Solid Edge part; units mm, degrees
sketch "Sketch1" plane through (0, 0, 0) normal (0, 0, 1) x (1, 0, 0)
  circle A0 centre (0, 0) radius 11
extrude "Protrusion1" add sketch "Sketch1" along normal blind 28
sketch "Sketch2" plane through (0, 0, 28) normal (0, 0, 1) x (1, 0, 0)
  circle A0 centre (0, 0) radius 19
extrude "ExtrudedProtrusion_2" add sketch "Sketch2" along normal blind 4
sketch "Sketch3" plane through (0, 0, 32) normal (0, 0, 1) x (1, 0, 0)
  line L0 (14, 14) -> (14, -14)
  line L1 (14, -14) -> (-14, -14)
  line L2 (-14, -14) -> (-14, 14)
  line L3 (-14, 14) -> (14, 14)
extrude "ExtrudedProtrusion_3" add sketch "Sketch3" along normal blind 7.5
sketch "Sketch4" plane through (0, 0, 39.5) normal (0, 0, 1) x (1, 0, 0)
  circle A0 centre (0, 0) radius 7
extrude "ExtrudedProtrusion_4" add sketch "Sketch4" along normal blind 20
sketch "Sketch5" plane through (0, 0, 59.5) normal (0, 0, 1) x (1, 0, 0)
  line L0 (7, -25) -> (7, 7)
  line L1 (7, 7) -> (-7, 7)
  line L2 (-7, 7) -> (-7, -25)
  line L3 (-7, -25) -> (7, -25)
extrude "ExtrudedProtrusion_5" add sketch "Sketch5" against normal blind 3.5
sketch "Sketch6" plane through (0, -9, 59.5) normal (0, 0, 1) x (1, 0, 0)
  circle A0 centre (0, 9) radius 5
  circle A1 centre (0, 9) radius 4
extrude "ExtrudedProtrusion_6" add sketch "Sketch6" along normal blind 10
sketch "Sketch7" plane through (0, -12.5, 56) normal (0, 0, -1) x (0, -1, 0)
  line L0 (-5.4984, 7) -> (-5.4984, -7)
  line L1 (-5.4984, -7) -> (-19.5, -7)
  line L2 (-19.5, -7) -> (-19.5, 7)
  line L3 (-19.5, 7) -> (-5.4984, 7)
extrude "Protrusion2" add sketch "Sketch7" along normal blind 12
sketch "Sketch8" plane through (7, -9, 51.75) normal (1, 0, 0) x (0, 1, 0)
  circle A0 centre (9, -4.5) radius 6.75
extrude "ExtrudedProtrusion_10" add sketch "Sketch8" against normal blind 26
sketch "Sketch9" plane through (-19, 0, 47.25) normal (-1, 0, 0) x (0, -1, 0)
  circle A0 centre (0, 0) radius 10.5
extrude "ExtrudedProtrusion_11" add sketch "Sketch9" along normal blind 15
sketch "Sketch10" plane through (-34, 0, 47.25) normal (-1, 0, 0) x (0, -1, 0)
  circle A0 centre (0, 0) radius 8.5
extrude "ExtrudedCutout_1" cut sketch "Sketch10" against normal blind 12.1174
sketch "Sketch11" plane through (0, 0, 0) normal (0, 0, -1) x (-1, 0, 0)
  circle A0 centre (0, 0) radius 10
extrude "ExtrudedCutout_2" cut sketch "Sketch11" against normal blind 35.1549
sketch "Sketch12" plane through (0, -9, 59.5) normal (0, 0, 1) x (1, 0, 0)
  circle A0 centre (0, 9) radius 4
extrude "Cutout1" cut sketch "Sketch12" against normal blind 106.077
sketch "Sketch13" plane through (-21.8826, 0, 47.25) normal (-1, 0, 0) x (0, -1, 0)
  circle A0 centre (0, 0) radius 4
extrude "ExtrudedCutout_4" cut sketch "Sketch13" against normal blind 21.2558
CAD build for the part. Positions are in the model's coordinates, mm. A direction names the side the tool comes from. Give positions to 0.01 mm unless a question says otherwise; leave off trailing zeros. Order: outer loops, then holes, each group sorted by start corner. A loop starts at its lowest first (then second) coordinate and runs counter-clockwise, first axis right, second up. Notation, with made-up numbers: (69, -29.75) - (96, -29.75) arc R22 ccw to (96, 0.25) - close; hole circle Ø4 at (49.25, -19). An arc over 180 degrees is marked (long way). Write each question's results on one line, items separated by ' | '.
1. Probe L1, parallel to Y at x = 0, z = 50; L2, parallel to Z at x = -26.25, y = 0; L3, parallel to Z at x = -18.5, y = 2. List the from-to ranges inside material, lowest first. Write a range as from..to.
Calculated:
L1: y = -7..-4, 4..7 | L2: z = 36.75..38.75, 55.75..57.75 | L3: z = 28..32, 40.8..43.79, 50.71..53.7
2. Saw through at C-C on z = 24. List the corners of the cut face in (x, y).
Calculated:
outline: circle Ø22 at (0, 0); hole circle Ø20 at (0, 0)
3. 3-axis set-ups, long thin cutter, end or side, ignore diameter. For faces 5 (the face through (-2.38, 10.74, 13.8)), 6 (the face through (0, -16, 32)), 7 (the face through (3.763, -5.902, 41.219)): which of +Z, -Z, +X, -X, +Y, -Y reach the whole face in a straight line?
Calculated:
face 5: -Z | face 6: +X, -X, -Y | face 7: none
4. Pin check, flat tips, straight feed: pin 1 (5 mm diameter, centred on x = -15.5, z = 45.5, fed in from +Y); pin 2 (0.9 mm diameter, centred on x = 0, y = -6.5, fed in from -Z); pin 3 (0.9 mm diameter, centred on x = 13.5, y = -13, fed in from -Z); pin 4 (1.5 mm diameter, centred on y = -14, z = 62, fed in from -X). Stop position of each tip, or through.
Calculated:
pin 1: stops at y = 6.75 | pin 2: stops at z = 35.15 | pin 3: stops at z = 28 | pin 4: passes through
5. Saw through at A-A on x = -17.5. List the corners of the cut face in (y, z).
Calculated:
outline: (-7.4, 28) - (7.4, 28) - (7.4, 32) - (-7.4, 32) - close; circle Ø13.5 at (0, 47.25); hole circle Ø8 at (0, 47.25)
6. Saw through at B-B on x = -23. List the corners of the cut face in (y, z).
Calculated:
outline: circle Ø21 at (0, 47.25); hole circle Ø17 at (0, 47.25)
7. Pull direction Z, two halves, no side cores. Call faces 1 (the face through (16, 0, 32)), 2 (the face through (14, 0, 36)), 3 (the face through (-28, -4.6, 54.4)), 4 (the face through (8, -8, 28)): released by +Z, released by -Z, zero draft, split by the parting line, or undercut.
Calculated:
face 1: released by +Z | face 2: zero draft | face 3: undercut | face 4: released by -Z
